Work out the finished part from the listing and answer in its coordinate system (mm). Face numbers are marked on the shaded views. A direction names the side the tool comes from. Round coordinates to 2 decimals unless told otherwise and drop trailing zeros. Loops run counter-clockwise (first coordinate to the right, second up) from the corner with the lowest first, then second, coordinate; pieces in that order, holes last. Notation, with made-up numbers: (81, 37) -> (105, 37) arc R35 cw to (105, 70) -> close; hole circle Ø6 at (87.5, -31). An arc over 180 degrees is marked (long way). Use CSV: the item, a comma, the result in double quotes. Start each with the question number.
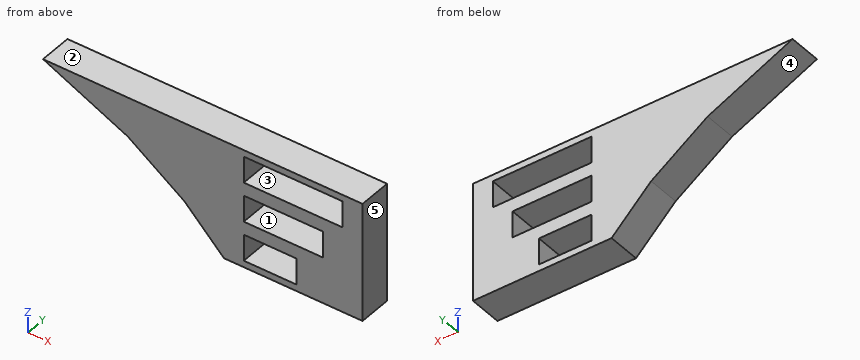
from build123d import *

# Parameters (mm, degrees)
F0_W     = 8
F0_H     = 4
F0_W_2   = 12
F0_W_3   = 15
F1_DEPTH = 5


with BuildPart() as f1:
    # F0 (on Front) → F1 (new body)
    with BuildSketch(Plane.XZ):
        Polygon((-3, 0), (0, 0), (18, 0), (18, 18), (0, 18), (-30.43593, 18), (-17.568888, 12), (-9, 6), align=None)
        with Locations((4, 3)):
            Rectangle(F0_W, F0_H, mode=Mode.SUBTRACT)
        with Locations((6, 9)):
            Rectangle(F0_W_2, F0_H, mode=Mode.SUBTRACT)
        with Locations((7.5, 15)):
            Rectangle(F0_W_3, F0_H, mode=Mode.SUBTRACT)
    extrude(amount=F1_DEPTH)


solid = f1.part
Q1. For a pull along X with two mould halves and no side action, classify the marked faces 3, 4 and 5 as pulls with the +X half, pulls with the -X half, needs draft (parallel to the pull), parting line crosses it, or undercut.
Q2. Each of these flat-tipped pins is pushed along its axis until it touches: pin 1 (1.2 mm diameter, centred on y = -3.5, z = 9, fed in from -X); pin 2 (1.5 mm diameter, centred on x = 6, y = -1.5, fed in from -Z); pin 3 (5 mm diameter, centred on x = -25.5, z = 11, fed in from +Y); pin 4 (2 mm diameter, centred on y = -1.5, z = 6.5, fed in from -X). Where does it stop, or does it pass through?
Q3. Section C-C, the plane y = -2.05 is taken. Write down the section's boundary in (x, z).
Q4. Section B-B, the plane z = 2.25 is taken. Write down the section's boundary in (x, y), and give its area (4 significant figures).
Q5. Which of the six approach directions +Z, -Z, +X, -X, +Y, -Y give full straight-line access (tool end or side, diameter ignored) to the marked faces 1 and 2?
Q6. Section A-A, the plane x = 8.5 is taken. Write down the section's boundary in (y, z).
Q7. Section D-D, the plane z = 9 is taken. Write down the section's boundary in (x, y).
Q8. Straight lines are drawn through the part: line 1 (Z direction, x = 10, y = -0.65); line 2 (Z direction, x = 7, y = -1.5); line 3 (Z direction, x = 13.5, y = -0.75). For each, find the intervals that lie inside material, in ascending order. Write a range as from..to.
Report:
1,face 3,"undercut"
1,face 4,"pulls with the -X half"
1,face 5,"pulls with the +X half"
2,pin 1,"stops at x = -14.14"
2,pin 2,"stops at z = 0"
2,pin 3,"passes through"
2,pin 4,"stops at x = -11.14"
3,outline,"(-30.44, 18) -> (-17.57, 12) -> (-9, 6) -> (-3, 0) -> (18, 0) -> (18, 18) -> close; hole (0, 1) -> (8, 1) -> (8, 5) -> (0, 5) -> close; hole (0, 7) -> (12, 7) -> (12, 11) -> (0, 11) -> close; hole (0, 13) -> (15, 13) -> (15, 17) -> (0, 17) -> close"
4,outline,"(-5.25, -5) -> (0, -5) -> (0, 0) -> (-5.25, 0) -> close; (8, -5) -> (18, -5) -> (18, 0) -> (8, 0) -> close"
4,area,"76.25 mm²"
5,face 1,"+Y, -Y"
5,face 2,"+Z, +X, -X, +Y, -Y"
6,outline,"(-5, 0) -> (0, 0) -> (0, 7) -> (-5, 7) -> close; (-5, 11) -> (0, 11) -> (0, 13) -> (-5, 13) -> close; (-5, 17) -> (0, 17) -> (0, 18) -> (-5, 18) -> close"
7,outline,"(-13.28, -5) -> (0, -5) -> (0, 0) -> (-13.28, 0) -> close; (12, -5) -> (18, -5) -> (18, 0) -> (12, 0) -> close"
8,line 1,"z = 0..7, 11..13, 17..18"
8,line 2,"z = 0..1, 5..7, 11..13, 17..18"
8,line 3,"z = 0..13, 17..18"
